Input: dimensioned drawing with shaded views. Units: mm. Origin: part minimum x, y, z. A direction names the side the tool comes from. Coordinates: 2 decimals unless noted, no trailing zeros. Order: outer loops, then holes, each group sorted by start corner. A loop starts at its lowest first (then second) coordinate and runs counter-clockwise, first axis right, second up.
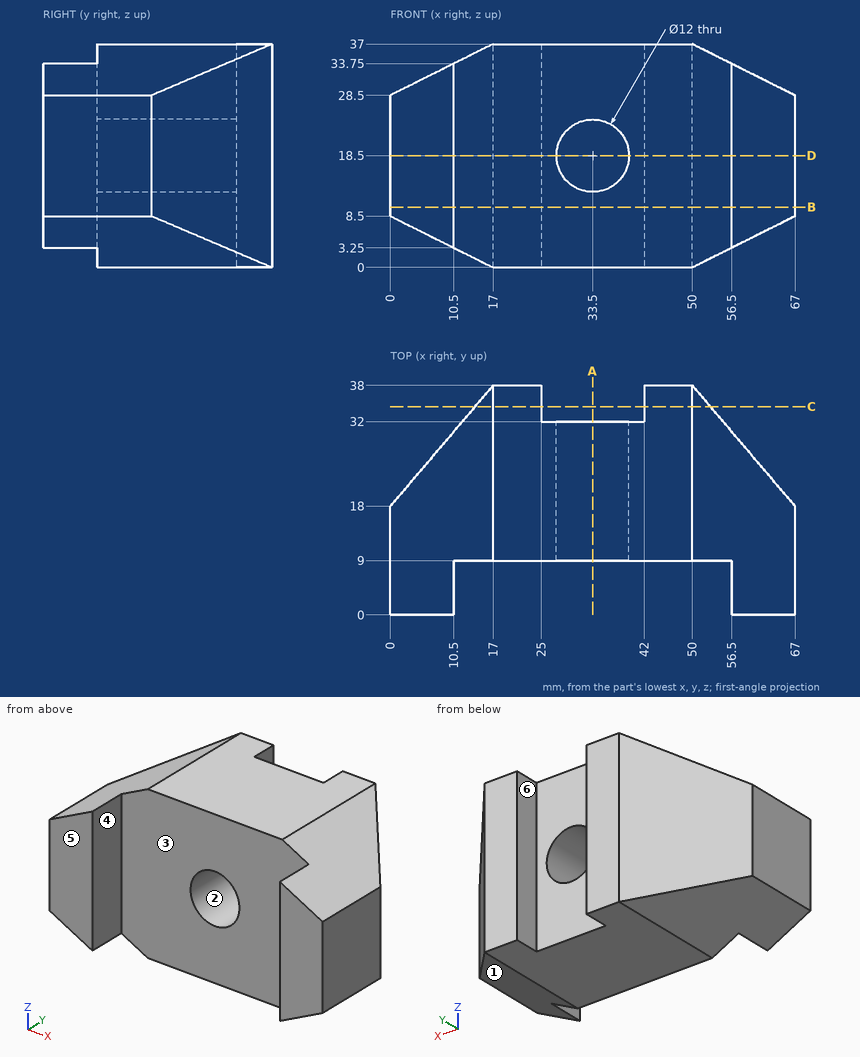
1. Section query D-D, the plane z = 18.5. Output: boundary loops of the cut face in (x, y), plus the area to 3 significant figures.
2. Contact query for flat-ended pins moving along their axis: P1, Ø11, axis at x = 22, z = 13.5, coming from the -Y side; P2, Ø6, axis at x = 40.5, y = 5.5, coming from the +Z side; P3, Ø5, axis at y = 22, z = 4, coming from the -X side; P4, Ø2, axis at y = 26.5, z = 30.5, coming from the +X side (3 decimals). Output: stop coordinate, or through.
3. Section query C-C, the plane y = 34.5. Output: boundary loops of the cut face in (x, z) (1 decimal).
4. Section query A-A, the plane x = 33.5. Output: boundary loops of the cut face in (y, z).
5. Material intervals for line 1 along X through (y, z) = (15.25, 18.5); line 2 along X through (y, z) = (21, 15.5); line 3 along Z through (x, y) = (33, 15), sorted ascending.
6. Section query B-B, the plane z = 10. Output: boundary loops of the cut face in (x, y), plus the area to 3 significant figures.
7. Draft query along Z for the marked faces 1, 2 and 3. Return one class per face: +Z half, -Z half, draft (parallel to the pull), parting line (faces both ways), or undercut.
8. Access query for the marked faces 4, 5 and 6. Directions: +Z, -Z, +X, -X, +Y, -Y. A direction counts if a zero-diameter tool reaches every point of the face in a straight line with its end or side. Return the directions, or none.
Answer key:
1. outline: (0, 0) - (10.5, 0) - (10.5, 9) - (27.5, 9) - (27.5, 32) - (25, 32) - (25, 38) - (17, 38) - (0, 18) - close; (39.5, 9) - (56.5, 9) - (56.5, 0) - (67, 0) - (67, 18) - (50, 38) - (42, 38) - (42, 32) - (39.5, 32) - close
1. area: 1,410 mm2
2. P1: stops at y = 9
2. P2: passes through
2. P3: stops at x = 4
2. P4: stops at x = 60.625
3. outline: (14, 1.5) - (17, 0) - (25, 0) - (25, 37) - (17, 37) - (14, 35.5) - close; (42, 0) - (50, 0) - (53, 1.5) - (53, 35.5) - (50, 37) - (42, 37) - close
4. outline: (9, 0) - (32, 0) - (32, 12.5) - (9, 12.5) - close; (9, 24.5) - (32, 24.5) - (32, 37) - (9, 37) - close
5. line 1: x = 0 to 27.5, 39.5 to 67
5. line 2: x = 2.55 to 28.3, 38.7 to 64.45
5. line 3: z = 0 to 12.52, 24.48 to 37
6. outline: (0, 0) - (10.5, 0) - (10.5, 9) - (56.5, 9) - (56.5, 0) - (67, 0) - (67, 18) - (50, 38) - (42, 38) - (42, 32) - (25, 32) - (25, 38) - (17, 38) - (0, 18) - close
6. area: 1,690 mm2
7. face 1: -Z half
7. face 2: undercut
7. face 3: draft
8. face 4: +Z, -Z, -Y
8. face 5: +Z, -Z, +X, -X, -Y
8. face 6: +Z, -Z, +Y
